Autodesk Inventor part; units mm, degrees
ref_plane "YZ Plane" through (0, 0, 0) normal (1, 0, 0) x (0, 1, 0)
ref_plane "XZ Plane" through (0, 0, 0) normal (0, 1, 0) x (-1, 0, 0)
ref_plane "XY Plane" through (0, 0, 0) normal (0, 0, 1) x (1, 0, 0)
sketch "Sketch1" plane through (0, 0, 0) normal (0, 0, 1) x (1, 0, 0)
  line L0 (5.644444, -5.644444) -> (-5.644444, -5.644444)
  line L1 (-5.644444, -5.644444) -> (-5.644444, 5.644444)
  line L2 (-5.644444, 5.644444) -> (5.644444, 5.644444)
  line L3 (5.644444, 5.644444) -> (5.644444, -5.644444)
  point P0 (0, 0)
  point P1 (0, 0)
  dimension "d0" = 11.28889
extrude "Extrusion1" add sketch "Sketch1" along normal blind 8.466667
ref_plane "Work Plane1" through (0, 5.644444, 8.466667) normal (-1, 0, 0) x (0, -1, 0)
sketch "Sketch2" plane through (0, 5.644444, 8.466667) normal (-1, 0, 0) x (0, -1, 0)
  line L0 (5.644444, -8.466667) -> (-2.822222, -8.466667)
  line L1 (0, -8.466667) -> (11.288889, -8.466667)
  line L2 (5.644444, -8.466667) -> (5.644444, -11.641667)
  arc A0 (-2.822222, -8.466667) -> (5.644444, -11.641667) centre (5.644444, 1.234722) ccw
  dimension "d3" = 8.46667
  dimension "d4" = 3.175
revolve "Revolution1" add sketch "Sketch2" angle 360 about axis through (0, 0, 0) along (0, 0, -1)
sketch "Sketch3" plane through (0, 0, 8.466667) normal (0, 0, 1) x (1, 0, 0)
  line L0 (-5.644444, -5.644444) -> (5.644444, -5.644444)
  line L1 (5.644444, -5.644444) -> (5.644444, 5.644444)
  line L2 (5.644444, 5.644444) -> (-5.644444, 5.644444)
  line L3 (-5.644444, 5.644444) -> (-5.644444, -5.644444)
  point P0 (0, 0)
extrude "Extrusion2" cut sketch "Sketch3" against normal up to surface (8.466667 mm away)
sketch "Sketch4" plane through (0, 0, 0) normal (0, 0, 1) x (1, 0, 0)
  circle A0 centre (0, 0) radius 4.233333
  dimension "d8" = 8.46667
extrude "Extrusion3" add sketch "Sketch4" along normal blind 11.288889 draft -10
sketch "Sketch5" plane through (0, 0, 0) normal (0, 0, 1) x (1, 0, 0)
  circle A0 centre (0, 0) radius 8.466667
  line L0 (8.466667, -4.888232) -> (0, -9.776465)
  line L1 (0, -9.776465) -> (-8.466667, -4.888232)
  line L2 (-8.466667, -4.888232) -> (-8.466667, 4.888232)
  line L3 (-8.466667, 4.888232) -> (0, 9.776465)
  line L4 (0, 9.776465) -> (8.466667, 4.888232)
  line L5 (8.466667, 4.888232) -> (8.466667, -4.888232)
  point P0 (0, 0)
  point P1 (0, 0)
  point P2 (8.466667, 0)
sketch "Sketch5 outline for Extrusion4" plane through (0, 0, 0) normal (0, 0, 1) x (1, 0, 0)
  line L0 (8.466667, 0) -> (8.466667, -4.888232)
  line L1 (8.466667, -4.888232) -> (0, -9.776465)
  line L2 (0, -9.776465) -> (-8.466667, -4.888232)
  line L3 (-8.466667, -4.888232) -> (-8.466667, 4.888232)
  line L4 (-8.466667, 4.888232) -> (0, 9.776465)
  line L5 (0, 9.776465) -> (8.466667, 4.888232)
  line L6 (8.466667, 4.888232) -> (8.466667, 0)
extrude "Extrusion4" add sketch "Sketch5 outline for Extrusion4" against normal blind 3.175 draft -10
properties part number "Driver Shaft Cap"
For this review, take the finished solid that the model builds, in its own axes (mm). A direction names the side the tool comes from. Round coordinates to 2 decimals unless told otherwise and drop trailing zeros. Loops run counter-clockwise (first coordinate to the right, second up) from the corner with the lowest first, then second, coordinate; pieces in that order, holes last.
(1) Clearance check with flat-ended pins moving along their axes: P1, Ø1, axis at x = 6, y = -7, coming from the +Z side; P2, Ø5, axis at y = 2.5, z = 7, coming from the -X side. State where each tip first meets the part, or that it passes through.
Returned:
P1: passes through
P2: stops at x = -3.23
(2) We need section A-A (y = 0). Give the boundary of the cut face in (x, z) (3 decimals).
Returned:
outline: (-8.467, 0) - (-7.907, -3.175) - (7.907, -3.175) - (8.467, 0) - (4.233, 0) - (2.243, 11.289) - (-2.243, 11.289) - (-4.233, 0) - close
(3) We need section B-B (z = -1.25). Give the boundary of the cut face in (x, y), plus the area to 3 significant figures.
Returned:
outline: (-8.25, -4.76) - (0, -9.52) - (8.25, -4.76) - (8.25, 4.76) - (0, 9.52) - (-8.25, 4.76) - close
area: 236 mm2
(4) We need section D-D (y = -5.25). Give the boundary of the cut face in (x, z) (3 decimals).
Returned:
outline: (-7.84, 0) - (-6.72, -3.175) - (6.72, -3.175) - (7.84, 0) - close
(5) Tool access review of faces 1 (the flat face through (-4, -2, 0)), 2 (the flat face through (8.19, 0.07, -1.57)): name each direction out of +Z, -Z, +X, -X, +Y, -Y from which nothing blocks a thin tool from reaching the whole face with its end or side.
Returned:
face 1: +Z
face 2: -Z, +X, +Y, -Y
(6) Wall thickness on line 1 along Z through (x, y) = (-6.5, 0) (3 decimals); line 2 along Y through (x, z) = (0.5, -1.75); line 3 along Y through (x, z) = (-1, 2.75): over which ranges is each line inside the solid? List them lowest first.
Returned:
line 1: z = -3.175 to 0
line 2: y = -9.13 to 9.13
line 3: y = -3.61 to 3.61
(7) We need section C-C (x = 6). Give the boundary of the cut face in (y, z) (3 decimals), plus the area to 3 significant figures.
Returned:
outline: (-6.312, 0) - (-5.666, -3.175) - (5.666, -3.175) - (6.312, 0) - close
area: 38.0 mm2
